```python
from build123d import *

# Parameters (mm, degrees)
ESTRUSIONE_ESTRUSIONE1_DEPTH = 10
SCHIZZO6_R                   = 11
TAGLIO_ESTRUSIONE4_DEPTH     = 7
SCHIZZO7_R                   = 4
TAGLIO_ESTRUSIONE5_DEPTH     = 4
SMUSSO2_SIZE                 = 10
SCHIZZO8_W                   = 20
SCHIZZO8_H                   = 4
ESTRUSIONE_ESTRUSIONE3_DEPTH = 15
SCHIZZO9_R                   = 2.5
TAGLIO_ESTRUSIONE6_DEPTH     = 35
RACCORDO1_R                  = 2
SCHIZZO10_R                  = 2
TAGLIO_ESTRUSIONE7_DEPTH     = 10


with BuildPart() as part:
    # Schizzo1 → Estrusione-Estrusione1 (new body)
    with BuildSketch(Plane.XY):
        Polygon((-10, -47.5), (10, -47.5), (10, -27.5), (21, -27.5), (21, 27.5), (-21, 27.5), (-21, -27.5), (-10, -27.5), align=None)
    extrude(amount=ESTRUSIONE_ESTRUSIONE1_DEPTH)

    # Schizzo6 → Taglio-Estrusione4 (cut)
    with BuildSketch(Plane.XY.offset(10)):
        Circle(SCHIZZO6_R)
    extrude(amount=-TAGLIO_ESTRUSIONE4_DEPTH, mode=Mode.SUBTRACT)

    # Schizzo7 → Taglio-Estrusione5 (cut, through all)
    with BuildSketch(Plane.XY.offset(3)):
        Circle(SCHIZZO7_R)
    extrude(amount=-TAGLIO_ESTRUSIONE5_DEPTH, mode=Mode.SUBTRACT)

    # Smusso2
    smusso2_edges = [part.edges().sort_by_distance(p)[0] for p in [
        (21, -27.5, 5),
        (-21, -27.5, 5),
        (-21, 27.5, 5),
        (21, 27.5, 5),
    ]]
    chamfer(smusso2_edges, length=SMUSSO2_SIZE)

    # Schizzo8 → Estrusione-Estrusione3 (add)
    with BuildSketch(Plane(origin=(0, 0, 0), x_dir=(-1, 0, 0), z_dir=(0, 0, -1))):
        with Locations((0, -45.5)):
            Rectangle(SCHIZZO8_W, SCHIZZO8_H)
    extrude(amount=ESTRUSIONE_ESTRUSIONE3_DEPTH)

    # Schizzo9 → Taglio-Estrusione6 (cut)
    with BuildSketch(Plane(origin=(0, -43.5, 0), x_dir=(1, 0, 0), z_dir=(0, 1, 0))):
        with Locations((0, 7.5)):
            Circle(SCHIZZO9_R)
    extrude(amount=-TAGLIO_ESTRUSIONE6_DEPTH, mode=Mode.SUBTRACT)

    # Raccordo1
    raccordo1_edges = [part.edges().sort_by_distance(p)[0] for p in [
        (0, -43.5, 0),
        (10, -45.5, -15),
        (-10, -45.5, -15),
    ]]
    fillet(raccordo1_edges, radius=RACCORDO1_R)

    # Schizzo10 → Taglio-Estrusione7 (cut)
    with BuildSketch(Plane(origin=(0, 0, 0), x_dir=(-1, 0, 0), z_dir=(0, 0, -1))):
        with Locations((0, -37.5)):
            Circle(SCHIZZO10_R)
    extrude(amount=-TAGLIO_ESTRUSIONE7_DEPTH, mode=Mode.SUBTRACT)


solid = part.part
```
Here's how the part is built. I have some questions about the finished solid (model axes, mm). A direction names the side the tool comes from. Round coordinates to 2 decimals unless told otherwise and drop trailing zeros. Write each loop counter-clockwise with the first axis right and the second up, starting at its lowest first coordinate (ties: lowest second). Pieces come first, ordered by that corner, then holes.
Q1. Please list where these lines run through material, in increasing order: probe 1 along Y at (x, z) = (0, 4.75); probe 2 along Y at (x, z) = (0, 2.5); probe 3 along Z at (x, y) = (0, -46).
Q2. If we section it at A-A on z = -7.5: Write out the boundary of the cut face in (x, y).
Q3. If we mould it in two halves opening along Z, with no side actions, what happens to faces 1 (the cylindrical face through (-0.14, -42.93, -0.6)), 2 (the cylindrical face through (-2.38, -10.74, 6.55)), 3 (the flat face through (9, -9, 10)), 4 (the cylindrical face through (-0.54, -45.47, -5.06))? For each: +Z half, -Z half, draft (parallel to the pull), parting line (faces both ways), or undercut.
Q4. Will these pins go through, and if not, where does the flat tip stop? P1, Ø24, axis at x = 0, y = -2, coming from the +Z side; P2, Ø8, axis at x = 0, z = -7.5, coming from the +Y side; P3, Ø20, axis at x = 0, y = 0, coming from the -Z side; P4, Ø0.8, axis at x = 10.5, z = 3, coming from the -Y side.
Q5. If we section it at C-C on y = 0: Write out the boundary of the cut face in (x, z), plus the area to 3 significant figures.
Q6. Which directions (+Z, -Z, +X, -X, +Y, -Y) give clear straight access to the entire face, cutting with the end or side of a thin tool? Please do faces 5 (the flat face through (2, -43.5, -10)), 6 (the flat face through (-16.1, -22.4, 4.9)), 7 (the flat face through (10, -40, 4)).
Q7. If we section it at D-D on z = 5.5: Write out the boundary of the cut face in (x, y), plus the area to 3 significant figures.
Q8. If we section it at B-B on x = 0: Write out the boundary of the cut face in (y, z), plus the area to 3 significant figures.
Answer below:
1. probe 1: y = -47.5 to -39.5, -35.5 to -11, 11 to 27.5
1. probe 2: y = -47.5 to -39.5, -35.5 to -4, 4 to 27.5
1. probe 3: z = -15 to -10, -5 to 10
2. outline: (-10, -47.5) - (-2.5, -47.5) - (-2.5, -43.5) - (-10, -43.5) - close; (2.5, -47.5) - (10, -47.5) - (10, -43.5) - (2.5, -43.5) - close
3. face 1: -Z half
3. face 2: draft
3. face 3: +Z half
3. face 4: undercut
4. P1: stops at z = 10
4. P2: stops at y = -43.5
4. P3: stops at z = 0
4. P4: stops at y = -27.5
5. outline: (-21, 0) - (-4, 0) - (-4, 3) - (-11, 3) - (-11, 10) - (-21, 10) - close; (4, 0) - (21, 0) - (21, 10) - (11, 10) - (11, 3) - (4, 3) - close
5. area: 242 mm2
6. face 5: -Z, +X, -X, +Y
6. face 6: +Z, -Z, -X, -Y
6. face 7: +Z, -Z, +X, -Y
7. outline: (-21, -17.5) - (-11, -27.5) - (-10, -27.5) - (-10, -47.5) - (10, -47.5) - (10, -27.5) - (11, -27.5) - (21, -17.5) - (21, 17.5) - (11, 27.5) - (-11, 27.5) - (-21, 17.5) - close; hole circle Ø22 at (0, 0); hole circle Ø4 at (0, -37.5)
7. area: 2,120 mm2
8. outline: (-47.5, -15) - (-43.5, -15) - (-43.5, -10) - (-47.5, -10) - close; (-47.5, -5) - (-43.5, -5) - (-43.5, -2) arc R2 cw to (-41.5, 0) - (-39.5, 0) - (-39.5, 10) - (-47.5, 10) - close; (-35.5, 0) - (-4, 0) - (-4, 3) - (-11, 3) - (-11, 10) - (-35.5, 10) - close; (4, 0) - (27.5, 0) - (27.5, 10) - (11, 10) - (11, 3) - (4, 3) - close
8. area: 573 mm2
